```python
from build123d import *

# Parameters (mm, degrees)
F0_W     = 64
F0_H     = 89
F0_W_2   = 63.8
F0_H_2   = 88.8
F0_W_3   = 50
F0_H_3   = 10
F1_DEPTH = 3
F2_R     = 2


with BuildPart() as f1:
    # F0 (on Top) → F1 (new body)
    with BuildSketch(Plane.XY):
        with Locations((-32, 44.5)):
            Rectangle(F0_W, F0_H)
        with Locations((-32, 44.5)):
            Rectangle(F0_W_2, F0_H_2, mode=Mode.SUBTRACT)
        with Locations((-32, 44.5)):
            Rectangle(F0_W_2, F0_H_2)
        with Locations((-32, 10.5)):
            Rectangle(F0_W_3, F0_H_3, mode=Mode.SUBTRACT)
        with Locations((-32, 27.5)):
            Rectangle(F0_W_3, F0_H_3, mode=Mode.SUBTRACT)
        with Locations((-32, 44.5)):
            Rectangle(F0_W_3, F0_H_3, mode=Mode.SUBTRACT)
        with Locations((-32, 61.5)):
            Rectangle(F0_W_3, F0_H_3, mode=Mode.SUBTRACT)
        with Locations((-32, 78.5)):
            Rectangle(F0_W_3, F0_H_3, mode=Mode.SUBTRACT)
    extrude(amount=F1_DEPTH)

    # F2
    f2_edges = [f1.edges().sort_by_distance(p)[0] for p in [
        (-57, 10.5, 3),
        (-32, 15.5, 3),
        (-7, 10.5, 3),
        (-32, 5.5, 3),
        (-57, 27.5, 3),
        (-32, 32.5, 3),
        (-7, 27.5, 3),
        (-32, 22.5, 3),
        (-32, 49.5, 3),
        (-7, 44.5, 3),
        (-32, 39.5, 3),
        (-57, 44.5, 3),
        (-7, 61.5, 3),
        (-32, 56.5, 3),
        (-57, 61.5, 3),
        (-32, 66.5, 3),
        (-7, 78.5, 3),
        (-32, 73.5, 3),
        (-57, 78.5, 3),
        (-32, 83.5, 3),
        (-32, 0, 3),
        (0, 44.5, 3),
        (-32, 89, 3),
        (-64, 44.5, 3),
    ]]
    fillet(f2_edges, radius=F2_R)


solid = f1.part
```
The listing builds one solid part. Answer for the finished solid, in the listing's coordinates (mm). A direction names the side the tool comes from. Coordinates: 2 decimals unless noted, no trailing zeros. Write each loop counter-clockwise with the first axis right and the second up, starting at its lowest first coordinate (ties: lowest second). Pieces come first, ordered by that corner, then holes.
Q1. Which of the six approach directions +Z, -Z, +X, -X, +Y, -Y give full straight-line access (tool end or side, diameter ignored) to faces 1 (the cylindrical face through (-57.57, 61.6, 2.4)), 2 (the cylindrical face through (-31.55, 88.43, 2.4))?
Returned:
face 1: +Z
face 2: +Z, +X, -X, +Y
Q2. Section B-B, the plane z = 2.25 is taken. Write down the section's boundary in (x, y), then the cut area to 3 significant figures.
Returned:
outline: (-63.56, 0.44) - (-0.44, 0.44) - (-0.44, 88.56) - (-63.56, 88.56) - close; hole (-57.44, 5.06) - (-6.56, 5.06) - (-6.56, 15.94) - (-57.44, 15.94) - close; hole (-57.44, 22.06) - (-6.56, 22.06) - (-6.56, 32.94) - (-57.44, 32.94) - close; hole (-57.44, 39.06) - (-6.56, 39.06) - (-6.56, 49.94) - (-57.44, 49.94) - close; hole (-57.44, 56.06) - (-6.56, 56.06) - (-6.56, 66.94) - (-57.44, 66.94) - close; hole (-57.44, 73.06) - (-6.56, 73.06) - (-6.56, 83.94) - (-57.44, 83.94) - close
area: 2,800 mm2
Q3. The mould has two halves that part along X. Classify faces 3 (the cylindrical face through (-0.57, 45.12, 2.4)), 4 (the flat face through (-32, 55, 0)), 5 (the cylindrical face through (-31.62, 67.07, 2.4)): released by +X, released by -X, zero draft, split by the parting line, or undercut.
Returned:
face 3: released by +X
face 4: zero draft
face 5: undercut
Q4. Section A-A, the plane y = 80.5 is taken. Write down the section's boundary in (x, z), then the cut area to 3 significant figures.
Returned:
outline: (-64, 0) - (-57, 0) - (-57, 1) arc R2 ccw to (-59, 3) - (-62, 3) arc R2 ccw to (-64, 1) - close; (-7, 0) - (0, 0) - (0, 1) arc R2 ccw to (-2, 3) - (-5, 3) arc R2 ccw to (-7, 1) - close
area: 38.6 mm2
Q5. Section C-C, the plane x = -47.5 is taken. Give the number of separate pieces and of enclosed holes in the cut face, then the cut area to 3 significant figures.
Returned:
separate pieces: 6
enclosed holes: 0
area: 107 mm2
Q6. Find the intervals of material crossed by line 1 along Y through (x, z) = (-50, 1.15); line 2 along Y through (x, z) = (-26.5, 1.6); line 3 along X through (y, z) = (58, 0.4), in increasing order.
Returned:
line 1: y = 0.01 to 5.49, 15.51 to 22.49, 32.51 to 39.49, 49.51 to 56.49, 66.51 to 73.49, 83.51 to 88.99
line 2: y = 0.09 to 5.41, 15.59 to 22.41, 32.59 to 39.41, 49.59 to 56.41, 66.59 to 73.41, 83.59 to 88.91
line 3: x = -64 to -57, -7 to 0
